Part model, mm, in its own coordinate system. Coordinates: 2 decimals unless noted, no trailing zeros. Write each loop counter-clockwise with the first axis right and the second up, starting at its lowest first coordinate (ties: lowest second). Pieces come first, ordered by that corner, then holes. Notation, with made-up numbers: M -12,-20.5 L 12,-20.5 A22 cw 12,0.5 Z; hole C 36.25,82 d11. An arc over 180 degrees is marked long. Use a Markdown table: item, result. Add a question column.
Q1. Slice it at A-A on x = 2.2. Write the cut outline in (y, z).
Q2. Slice it at C-C on x = 3.5. Write the cut outline in (y, z).
Q3. Mould opens along Y. For faces 1 (the flat face through (1.98, 3.48, -1.97)), 2 (the flat face through (4, -1, -1)), 3 (the cylindrical face through (1.98, -0.03, 0.61)) say: released by +Y, released by -Y, zero draft, split by the parting line, or undercut.
Q4. Slice it at B-B on y = 0. Write the cut outline in (x, z).
Q5. Pin check, flat tips, straight feed: pin 1 Ø1.1 at (y, z) = (0, 0) entering from +X; pin 2 Ø1 at (x, y) = (1.5, 3) entering from +Z; pin 3 Ø1.5 at (x, z) = (2, 3) entering from +Y. Stop position of each tip, or through.
Q6. Wall check: L1, parallel to Z at x = 1.55, y = 0; L2, parallel to Y at x = 0.9, z = 0.5; L3, parallel to X at y = 2, z = 3.5. Give the ranges that are in metal, low to high. Write a range as from..to.
Autodesk Inventor part; units mm, degrees
ref_plane "Work Plane1" through (-8.8582, 0, 0) normal (0, -0.866, -0.5) x (1, 0, 0)
ref_plane "YZ Plane" through (0, 0, 0) normal (1, 0, 0) x (0, 1, 0)
ref_plane "XZ Plane" through (0, 0, 0) normal (0, 1, 0) x (-1, 0, 0)
sketch "Sketch1" plane through (0, 0, 0) normal (1, 0, 0) x (0, 1, 0)
  line L0 (-4.6188, 0) -> (-2.3094, 4)
  line L1 (-2.3094, 4) -> (2.3094, 4)
  line L2 (2.3094, 4) -> (4.6188, 0)
  line L3 (4.6188, 0) -> (2.3094, -4)
  line L4 (2.3094, -4) -> (-2.3094, -4)
  line L5 (-2.3094, -4) -> (-4.6188, 0)
  point P0 (0, 0)
  point P1 (0, 0)
  dimension "d0" = 9.2376
extrude "Body" add sketch "Sketch1" along normal blind 4
sketch "Sketch2" plane through (0, 0, 0) normal (0, 0, 1) x (1, 0, 0)
  line L0 (0, 2.3094) -> (0, 4.6188)
  line L1 (0, 4.6188) -> (4, 4.6188)
  line L2 (4, 2.3094) -> (4, 4.6188)
  line L3 (-0.16, 0) -> (0.96, 0)
  line L4 (0.7325, 4.6188) -> (0, 3.35)
  line L5 (3.2675, 4.6188) -> (4, 3.35)
  dimension "d3" = 30
  dimension "d4" = 30
  dimension "d5" = 6.7
  dimension "d6" = 6.7
revolve "Chamfer1" cut sketch "Sketch2" angle 360 about axis through (-10, 0, 0) along (1, 0, 0)
sketch "Sketch3" plane through (4, 0, 0) normal (1, 0, 0) x (0, 0, -1)
  arc A0 (-0.625, -1.0825) -> (0.625, -1.0825) centre (0, 0) ccw
hole "Thread" at (4, 0, 0) direction (-1, 0, 0) diameter 1.221 end through all
chamfer "Chamfer2" distance 0.433 angle 30 1 edges at (4, 0, 0.6105) measured on face at (4, 2.4029, -0.2918)
chamfer "Chamfer3" distance 0.433 angle 30 1 edges at (0, 0, 0.6105) measured on face at (0, 2.4029, -0.2918)
ref_plane "Work Plane1" through (-8.8582, 0, 0) normal (0, -0.866, -0.5) x (1, 0, 0)
equation "\"d0\" = 1.1547 * SW"
equation "\"d1\" = KOH"
equation "\"d3\" = ANG1"
equation "\"d4\" = ANG2"
equation "\"d5\" = SW0"
equation "\"d6\" = SW01"
equation "\"d8\" = -0.5 * GD1 + 0.5 * NND"
equation "\"d40\" = -0.5 * GD1 + 0.5 * NND"
equation "\"d10\" = -0.5 * GD1 + 0.5 * NND"
equation "\"d41\" = -0.5 * GD1 + 0.5 * NND"
equation "\"ANG1\" = 30deg"
equation "\"ANG2\" = 30deg"
equation "\"NND\" = 5"
equation "\"KOH\" = 4"
equation "\"SW\" = 8"
equation "\"SW0\" = 6.7"
equation "\"SW01\" = 6.7"
equation "\"GUL\" = 0.541266 * PTC"
equation "\"THREADDIA\" = 5"
equation "\"TOA\" = 30deg"
equation "\"PTC\" = 0.8"
equation "\"E0\" = 1.155 * SW"
equation "\"GAL\" = 0.541266 * PTC"
properties part number "DIN 555-5 - M5" material "Steel, Mild"
Recorded:
| question | item | result |
|---|---|---|
| 1 | outline | M -4.62,0 L -2.31,-4 L 2.31,-4 L 4.62,0 L 2.31,4 L -2.31,4 Z; hole C 0,0 d1.22 |
| 2 | outline | M -4.13,-0.85 L -2.8,-3.15 A4.22 ccw -1.33,-4 L 1.33,-4 A4.22 ccw 2.8,-3.15 L 4.13,-0.85 A4.22 ccw 4.13,0.85 L 2.8,3.15 A4.22 ccw 1.33,4 L -1.33,4 A4.22 ccw -2.8,3.15 L -4.13,0.85 A4.22 ccw Z; hole C 0,0 d1.22 |
| 3 | face 1 | released by +Y |
| 3 | face 2 | zero draft |
| 3 | face 3 | undercut |
| 4 | outline | M 0,-3.35 L 0.38,-4 L 3.62,-4 L 4,-3.35 L 4,-1.04 L 3.75,-0.61 L 0.25,-0.61 L 0,-1.04 Z; M 0,1.04 L 0.25,0.61 L 3.75,0.61 L 4,1.04 L 4,3.35 L 3.62,4 L 0.38,4 L 0,3.35 Z |
| 5 | pin 1 | through |
| 5 | pin 2 | z = 3.67 |
| 5 | pin 3 | y = 3.32 |
| 6 | L1 | -4..-0.61, 0.61..4 |
| 6 | L2 | -4.33..-0.35, 0.35..4.33 |
| 6 | L3 | 0.39..3.61 |
